Model file for the job. Use its own axes, mm. A direction names the side the tool comes from. Round coordinates to 2 decimals unless told otherwise and drop trailing zeros. Loops run counter-clockwise (first coordinate to the right, second up) from the corner with the lowest first, then second, coordinate; pieces in that order, holes last. Notation, with made-up numbers: M 5.5,-38 L 57.5,-38 A11 ccw 57.5,-25 Z; hole C 21.5,-28.75 d6. An arc over 180 degrees is marked long. Use a Markdown table: item, result. Add a question column.
Item 1: Wall check: L1, parallel to X at y = -3, z = 67.5; L2, parallel to Y at x = 7, z = 56; L3, parallel to Y at x = 2, z = 101.5. Give the ranges that are in metal, low to high. Write a range as from..to.
Item 2: Two-plate mould, pull along X, no slides. Class faces 5 (the flat face through (5, -2, 99)), 6 (the flat face through (30.3, -3.6, 200)), 7 (the flat face through (4, -3, 99)): +X half, -X half, draft (parallel to the pull), parting line (faces both ways), or undercut.
Item 3: Pin check, flat tips, straight feed: P1, Ø1.1, axis at y = -6, z = 164, coming from the -X side; P2, Ø1.1, axis at y = -6, z = 196.5, coming from the +X side; P3, Ø1.5, axis at x = 21.5, z = 89, coming from the +Y side. Stop position of each tip, or through.
Item 4: Tool access for faces 1 (the flat face through (7, -6, 200)), 2 (the flat face through (33, 0, 99)), 3 (the flat face through (2, 0, 99)), 4 (the flat face through (30, -2, 99)): list every direction of +Z, -Z, +X, -X, +Y, -Y with a clear straight run to the whole face (end or side of a thin tool).
Item 5: Saw through at B-B on z = 181.5. Write the cut outline in (x, y).
Item 6: Saw through at A-A on z = 14. Write the cut outline in (x, y), then the cut area to 3 significant figures.
Item 7: Saw through at C-C on x = 25. Write the cut outline in (y, z).
```python
from build123d import *

# Parameters (mm, degrees)
BOSS_EXTRUDE1_DEPTH = 200
CUT_EXTRUDE1_DEPTH  = 2


with BuildPart() as part:
    # Sketch1 → Boss-Extrude1 (new body)
    with BuildSketch(Plane.XY):
        with BuildLine():
            Line((0, 0), (0, 1))
            Line((0, 1), (4.2, 1))
            ThreePointArc((4.2, 1), (4.765685425, 0.765685425), (5, 0.2))
            Line((5, 0.2), (5, -4.7))
            ThreePointArc((5, -4.7), (5.234314575, -5.265685425), (5.8, -5.5))
            Line((5.8, -5.5), (29.2, -5.5))
            ThreePointArc((29.2, -5.5), (29.765685425, -5.265685425), (30, -4.7))
            Line((30, -4.7), (30, 0.2))
            ThreePointArc((30, 0.2), (30.234314575, 0.765685425), (30.8, 1))
            Line((30.8, 1), (35, 1))
            Line((35, 1), (35, 0))
            Line((35, 0), (31.8, 0))
            ThreePointArc((31.8, 0), (31.234314575, -0.234314575), (31, -0.8))
            Line((31, -0.8), (31, -5.7))
            ThreePointArc((31, -5.7), (30.765685425, -6.265685425), (30.2, -6.5))
            Line((30.2, -6.5), (4.8, -6.5))
            ThreePointArc((4.8, -6.5), (4.234314575, -6.265685425), (4, -5.7))
            Line((4, -5.7), (4, -0.8))
            ThreePointArc((4, -0.8), (3.765685425, -0.234314575), (3.2, 0))
            Line((3.2, 0), (0, 0))
        make_face()
    extrude(amount=BOSS_EXTRUDE1_DEPTH)

    # Sketch2 → Cut-Extrude1 (cut, through all)
    with BuildSketch(Plane(origin=(0, -5.5, 0), x_dir=(1, 0, 0), z_dir=(0, 1, 0))):
        with BuildLine():
            Line((17.4, -6.300946702), (17.6, -6.300946702))
            ThreePointArc((17.6, -6.300946702), (19.367766953, -7.033179749), (20.1, -8.800946702))
            Line((20.1, -8.800946702), (20.1, -28.800946702))
            ThreePointArc((20.1, -28.800946702), (19.367766953, -30.568713655), (17.6, -31.300946702))
            Line((17.6, -31.300946702), (17.4, -31.300946702))
            ThreePointArc((17.4, -31.300946702), (15.632233047, -30.568713655), (14.9, -28.800946702))
            Line((14.9, -28.800946702), (14.9, -8.800946702))
            ThreePointArc((14.9, -8.800946702), (15.632233047, -7.033179749), (17.4, -6.300946702))
        make_face()
        with BuildLine():
            Line((14.9, -44.800946702), (14.9, -64.800946702))
            ThreePointArc((14.9, -64.800946702), (15.632233047, -66.568713655), (17.4, -67.300946702))
            Line((17.4, -67.300946702), (17.6, -67.300946702))
            ThreePointArc((17.6, -67.300946702), (19.367766953, -66.568713655), (20.1, -64.800946702))
            Line((20.1, -64.800946702), (20.1, -44.800946702))
            ThreePointArc((20.1, -44.800946702), (19.367766953, -43.033179749), (17.6, -42.300946702))
            Line((17.6, -42.300946702), (17.4, -42.300946702))
            ThreePointArc((17.4, -42.300946702), (15.632233047, -43.033179749), (14.9, -44.800946702))
        make_face()
        with BuildLine():
            Line((14.9, -80.800946702), (14.9, -100.800946702))
            ThreePointArc((14.9, -100.800946702), (15.632233047, -102.568713655), (17.4, -103.300946702))
            Line((17.4, -103.300946702), (17.6, -103.300946702))
            ThreePointArc((17.6, -103.300946702), (19.367766953, -102.568713655), (20.1, -100.800946702))
            Line((20.1, -100.800946702), (20.1, -80.800946702))
            ThreePointArc((20.1, -80.800946702), (19.367766953, -79.033179749), (17.6, -78.300946702))
            Line((17.6, -78.300946702), (17.4, -78.300946702))
            ThreePointArc((17.4, -78.300946702), (15.632233047, -79.033179749), (14.9, -80.800946702))
        make_face()
        with BuildLine():
            Line((14.9, -116.800946702), (14.9, -136.800946702))
            ThreePointArc((14.9, -136.800946702), (15.632233047, -138.568713655), (17.4, -139.300946702))
            Line((17.4, -139.300946702), (17.6, -139.300946702))
            ThreePointArc((17.6, -139.300946702), (19.367766953, -138.568713655), (20.1, -136.800946702))
            Line((20.1, -136.800946702), (20.1, -116.800946702))
            ThreePointArc((20.1, -116.800946702), (19.367766953, -115.033179749), (17.6, -114.300946702))
            Line((17.6, -114.300946702), (17.4, -114.300946702))
            ThreePointArc((17.4, -114.300946702), (15.632233047, -115.033179749), (14.9, -116.800946702))
        make_face()
        with BuildLine():
            Line((14.9, -152.800946702), (14.9, -172.800946702))
            ThreePointArc((14.9, -172.800946702), (15.632233047, -174.568713655), (17.4, -175.300946702))
            Line((17.4, -175.300946702), (17.6, -175.300946702))
            ThreePointArc((17.6, -175.300946702), (19.367766953, -174.568713655), (20.1, -172.800946702))
            Line((20.1, -172.800946702), (20.1, -152.800946702))
            ThreePointArc((20.1, -152.800946702), (19.367766953, -151.033179749), (17.6, -150.300946702))
            Line((17.6, -150.300946702), (17.4, -150.300946702))
            ThreePointArc((17.4, -150.300946702), (15.632233047, -151.033179749), (14.9, -152.800946702))
        make_face()
        with BuildLine():
            Line((14.9, -188.800946702), (14.9, -208.800946702))
            ThreePointArc((14.9, -208.800946702), (15.632233047, -210.568713655), (17.4, -211.300946702))
            Line((17.4, -211.300946702), (17.6, -211.300946702))
            ThreePointArc((17.6, -211.300946702), (19.367766953, -210.568713655), (20.1, -208.800946702))
            Line((20.1, -208.800946702), (20.1, -188.800946702))
            ThreePointArc((20.1, -188.800946702), (19.367766953, -187.033179749), (17.6, -186.300946702))
            Line((17.6, -186.300946702), (17.4, -186.300946702))
            ThreePointArc((17.4, -186.300946702), (15.632233047, -187.033179749), (14.9, -188.800946702))
        make_face()
    extrude(amount=-CUT_EXTRUDE1_DEPTH, mode=Mode.SUBTRACT)


solid = part.part
```
Entries:
| question | item | result |
|---|---|---|
| 1 | L1 | 4..5, 30..31 |
| 1 | L2 | -6.5..-5.5 |
| 1 | L3 | 0..1 |
| 2 | face 5 | undercut |
| 2 | face 6 | draft |
| 2 | face 7 | -X half |
| 3 | P1 | x = 4 |
| 3 | P2 | x = 31 |
| 3 | P3 | y = -5.5 |
| 4 | face 1 | +Z, +X, -X, +Y, -Y |
| 4 | face 2 | +Z, -Z, +X, -Y |
| 4 | face 3 | +Z, -Z, -X, -Y |
| 4 | face 4 | +Z, -Z, +Y |
| 5 | outline | M 0,0 L 3.2,0 A0.8 cw 4,-0.8 L 4,-5.7 A0.8 ccw 4.8,-6.5 L 30.2,-6.5 A0.8 ccw 31,-5.7 L 31,-0.8 A0.8 cw 31.8,0 L 35,0 L 35,1 L 30.8,1 A0.8 ccw 30,0.2 L 30,-4.7 A0.8 cw 29.2,-5.5 L 5.8,-5.5 A0.8 cw 5,-4.7 L 5,0.2 A0.8 ccw 4.2,1 L 0,1 Z |
| 6 | outline | M 0,0 L 3.2,0 A0.8 cw 4,-0.8 L 4,-5.7 A0.8 ccw 4.8,-6.5 L 14.9,-6.5 L 14.9,-5.5 L 5.8,-5.5 A0.8 cw 5,-4.7 L 5,0.2 A0.8 ccw 4.2,1 L 0,1 Z; M 20.1,-6.5 L 30.2,-6.5 A0.8 ccw 31,-5.7 L 31,-0.8 A0.8 cw 31.8,0 L 35,0 L 35,1 L 30.8,1 A0.8 ccw 30,0.2 L 30,-4.7 A0.8 cw 29.2,-5.5 L 20.1,-5.5 Z |
| 6 | area | 42.8 mm2 |
| 7 | outline | M -6.5,0 L -5.5,0 L -5.5,200 L -6.5,200 Z |
